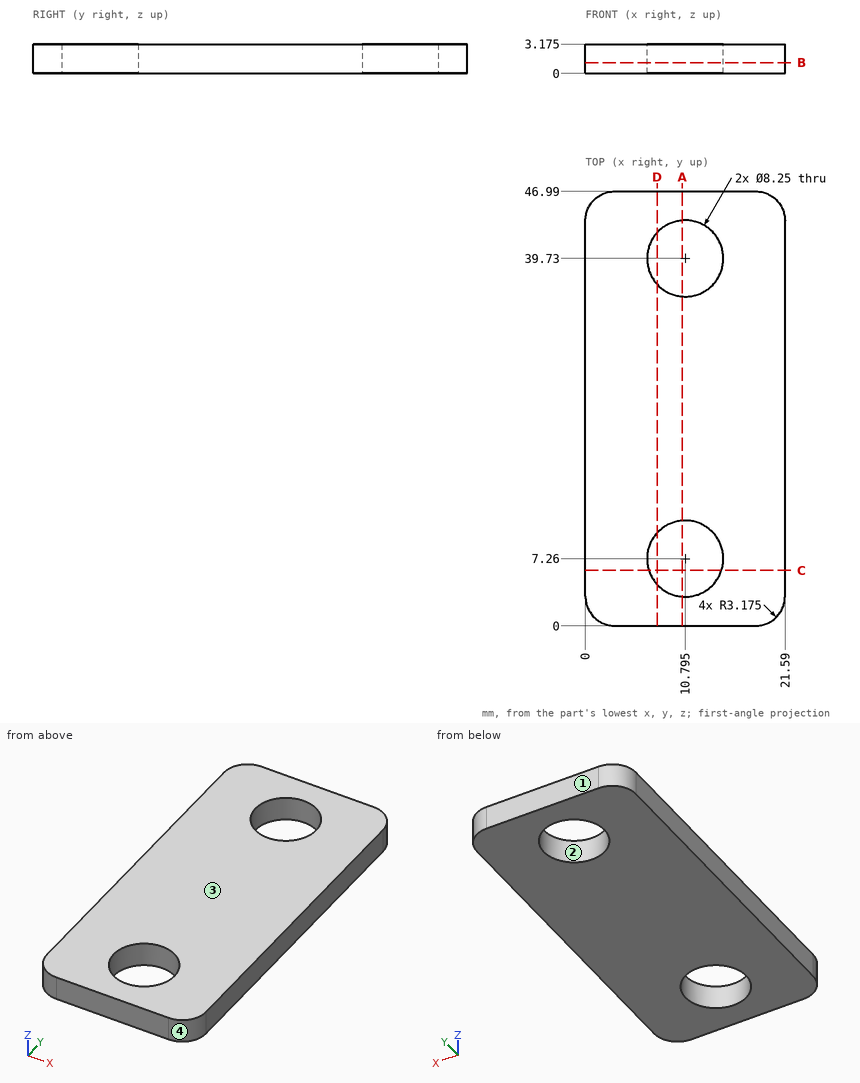
Study the drawing (mm; zero at the part's minimum x, y, z) and answer. Give positions to 0.01 mm unless a question says otherwise; leave off trailing zeros. Write each loop counter-clockwise with the first axis right and the second up, starting at its lowest first coordinate (ties: lowest second). Pieces come first, ordered by that corner, then holes. Notation, with made-up numbers: (8, -24) - (45, -24) arc R22 cw to (45, 8) - close; hole circle Ø4 at (-29.75, 53.5). An arc over 180 degrees is marked (long way). One line per question, with ' | ' between items. Start each with the question number.
1. Section D-D, the plane x = 7.75 is taken. Determine the outline of the cut face in (y, z) (1 decimal), then the cut area to 3 significant figures.
2. Section B-B, the plane z = 1.15 is taken. Count the separate pieces of the cut face and the enclosed holes in it, then the cut area to 3 significant figures.
3. Section C-C, the plane y = 6 is taken. Determine the outline of the cut face in (x, z) (1 decimal), then the cut area to 3 significant figures.
4. Straight lines are drawn through the part: line 1 (Y direction, x = 9, z = 2); line 2 (Y direction, x = 10, z = 2.55); line 3 (X direction, y = 36.5, z = 1.95). For each, find the intervals that lie inside material, in ascending order.
5. Section A-A, the plane x = 10.5 is taken. Determine the outline of the cut face in (y, z) (1 decimal).
6. Given P1, Ø1.5, axis at x = 8.5, z = 2.5, coming from the -Y side, flat-ended and moving along its own axis, determine where the tip first touches the part or whether it passes through.
7. Determine the mould class of the marked faces 1, 2, 3 and 4 for opening direction Y: +Y half, -Y half, draft (parallel to the pull), parting line (faces both ways), or undercut.
Result:
1) outline: (0, 0) - (4.5, 0) - (4.5, 3.2) - (0, 3.2) - close; (10, 0) - (36.9, 0) - (36.9, 3.2) - (10, 3.2) - close; (42.5, 0) - (47, 0) - (47, 3.2) - (42.5, 3.2) - close | area: 114 mm2
2) separate pieces: 1 | enclosed holes: 2 | area: 899 mm2
3) outline: (0, 0) - (6.9, 0) - (6.9, 3.2) - (0, 3.2) - close; (14.7, 0) - (21.6, 0) - (21.6, 3.2) - (14.7, 3.2) - close | area: 43.6 mm2
4) line 1: y = 0 to 3.55, 10.97 to 36.02, 43.44 to 46.99 | line 2: y = 0 to 3.21, 11.31 to 35.68, 43.78 to 46.99 | line 3: x = 0 to 8.23, 13.36 to 21.59
5) outline: (0, 0) - (3.1, 0) - (3.1, 3.2) - (0, 3.2) - close; (11.4, 0) - (35.6, 0) - (35.6, 3.2) - (11.4, 3.2) - close; (43.8, 0) - (47, 0) - (47, 3.2) - (43.8, 3.2) - close
6) P1: stops at y = 0
7) face 1: +Y half | face 2: undercut | face 3: draft | face 4: -Y half
